```python
from build123d import *

# Parameters (mm, degrees)
SKETCH1_R           = 177.8
BOSS_EXTRUDE1_DEPTH = 6.35
SKETCH2_R           = 2.286
SKETCH2_W           = 38.1
SKETCH2_H           = 127
SKETCH2_W_2         = 6.35
SKETCH2_H_2         = 25.4
CUT_EXTRUDE1_DEPTH  = 252.527339468


with BuildPart() as part:
    # Sketch1 → Boss-Extrude1 (new body)
    with BuildSketch(Plane(origin=(0, 0, 0), x_dir=(1, 0, 0), z_dir=(0, 1, 0))):
        with Locations(Location((0, 0, 0), (0, 0, 270))):
            Circle(SKETCH1_R)
    extrude(amount=BOSS_EXTRUDE1_DEPTH)

    # Sketch2 → Cut-Extrude1 (cut, through all)
    with BuildSketch(Plane(origin=(0, 6.35, 0), x_dir=(1, 0, 0), z_dir=(0, 1, 0))):
        with Locations(Location((-149.225, 25.4, 0), (0, 0, 270))):
            Circle(SKETCH2_R)
        with Locations(Location((-149.225, -25.4, 0), (0, 0, 90))):
            Circle(SKETCH2_R)
        with Locations(Location((-92.075, -25.4, 0), (0, 0, 270))):
            Circle(SKETCH2_R)
        with Locations(Location((-92.075, 25.4, 0), (0, 0, 90))):
            Circle(SKETCH2_R)
        with Locations(Location((92.075, 25.4, 0), (0, 0, 270))):
            Circle(SKETCH2_R)
        with Locations(Location((92.075, -25.4, 0), (0, 0, 90))):
            Circle(SKETCH2_R)
        with Locations(Location((149.225, -25.4, 0), (0, 0, 270))):
            Circle(SKETCH2_R)
        with Locations(Location((149.225, 25.4, 0), (0, 0, 90))):
            Circle(SKETCH2_R)
        with Locations((-120.65, 0)):
            Rectangle(SKETCH2_W, SKETCH2_H)
        with Locations((-149.225, 50.8)):
            Rectangle(SKETCH2_W_2, SKETCH2_H_2)
        with Locations((-149.225, 0)):
            Rectangle(SKETCH2_W_2, SKETCH2_H_2)
        with Locations((-149.225, -50.8)):
            Rectangle(SKETCH2_W_2, SKETCH2_H_2)
        with Locations((-92.075, -50.8)):
            Rectangle(SKETCH2_W_2, SKETCH2_H_2)
        with Locations((-92.075, 0)):
            Rectangle(SKETCH2_W_2, SKETCH2_H_2)
        with Locations((-92.075, 50.8)):
            Rectangle(SKETCH2_W_2, SKETCH2_H_2)
        with Locations((92.075, 50.8)):
            Rectangle(SKETCH2_W_2, SKETCH2_H_2)
        with Locations((92.075, 0)):
            Rectangle(SKETCH2_W_2, SKETCH2_H_2)
        with Locations((92.075, -50.8)):
            Rectangle(SKETCH2_W_2, SKETCH2_H_2)
        with Locations((149.225, -50.8)):
            Rectangle(SKETCH2_W_2, SKETCH2_H_2)
        with Locations((149.225, 0)):
            Rectangle(SKETCH2_W_2, SKETCH2_H_2)
        with Locations((149.225, 50.8)):
            Rectangle(SKETCH2_W_2, SKETCH2_H_2)
        with Locations((120.65, 0)):
            Rectangle(SKETCH2_W, SKETCH2_H)
    extrude(amount=-CUT_EXTRUDE1_DEPTH, mode=Mode.SUBTRACT)


solid = part.part
```
Part model, mm, in its own coordinate system. Round coordinates to 2 decimals unless told otherwise and drop trailing zeros. Write each loop counter-clockwise with the first axis right and the second up, starting at its lowest first coordinate (ties: lowest second). Pieces come first, ordered by that corner, then holes.
Item 1: Drop flat-ended pins along their axis: pin 1 Ø1.9 at (y, z) = (2.5, -54) entering from +X; pin 2 Ø2 at (y, z) = (1, 62.5) entering from +X (3 decimals); pin 3 Ø1.9 at (y, z) = (4, -46.5) entering from +X. Give the stop position or say it passes through.
Results:
pin 1: stops at x = 169.7
pin 2: stops at x = 166.825
pin 3: stops at x = 171.87
Item 2: Probe L1, parallel to Z at x = -148, y = 2.75; L2, parallel to Z at x = 139, y = 5.25; L3, parallel to Z at x = -104, y = 1. List the from-to ranges inside material, lowest first.
Results:
L1: z = -98.53 to -63.5, -38.1 to -27.33, -23.47 to -12.7, 12.7 to 23.47, 27.33 to 38.1, 63.5 to 98.53
L2: z = -110.87 to -63.5, 63.5 to 110.87
L3: z = -144.21 to -63.5, 63.5 to 144.21
Item 3: Cut at C-C, the plane y = 3.25. Count the separate pieces of the cut face and the enclosed holes in it, plus the area to 3 significant figures.
Results:
separate pieces: 1
enclosed holes: 22
area: 87,600 mm2
Item 4: Cut at D-D, the plane z = -123.5. Give the cut face in (x, y).
Results:
outline: (-127.91, 0) - (127.91, 0) - (127.91, 6.35) - (-127.91, 6.35) - close
Item 5: Cut at A-A, the plane z = 0. Give the cut face in (x, y).
Results:
outline: (-177.8, 0) - (-152.4, 0) - (-152.4, 6.35) - (-177.8, 6.35) - close; (-146.05, 0) - (-139.7, 0) - (-139.7, 6.35) - (-146.05, 6.35) - close; (-101.6, 0) - (-95.25, 0) - (-95.25, 6.35) - (-101.6, 6.35) - close; (-88.9, 0) - (88.9, 0) - (88.9, 6.35) - (-88.9, 6.35) - close; (95.25, 0) - (101.6, 0) - (101.6, 6.35) - (95.25, 6.35) - close; (139.7, 0) - (146.05, 0) - (146.05, 6.35) - (139.7, 6.35) - close; (152.4, 0) - (177.8, 0) - (177.8, 6.35) - (152.4, 6.35) - close
Item 6: Cut at B-B, the plane z = 54. Give the cut face in (x, y).
Results:
outline: (-169.4, 0) - (-152.4, 0) - (-152.4, 6.35) - (-169.4, 6.35) - close; (-146.05, 0) - (-139.7, 0) - (-139.7, 6.35) - (-146.05, 6.35) - close; (-101.6, 0) - (-95.25, 0) - (-95.25, 6.35) - (-101.6, 6.35) - close; (-88.9, 0) - (88.9, 0) - (88.9, 6.35) - (-88.9, 6.35) - close; (95.25, 0) - (101.6, 0) - (101.6, 6.35) - (95.25, 6.35) - close; (139.7, 0) - (146.05, 0) - (146.05, 6.35) - (139.7, 6.35) - close; (152.4, 0) - (169.4, 0) - (169.4, 6.35) - (152.4, 6.35) - close
